For this review, take the finished solid that the model builds, in its own axes (mm). A direction names the side the tool comes from. Coordinates: 2 decimals unless noted, no trailing zeros. Loops run counter-clockwise (first coordinate to the right, second up) from the corner with the lowest first, then second, coordinate; pieces in that order, holes last. Notation, with made-up numbers: (10, 14.25) - (16, 14.25) arc R12 ccw to (16, 23.25) - close; hole circle Ø5 at (-13, -8). An arc over 180 degrees is marked (long way). Answer as a JSON object with one key per item and string values. Group by question number.
Item 1: To check wall thickness, follow line 1 (X direction, y = -18.5, z = 2.5); line 2 (Y direction, x = 21.5, z = -3); line 3 (Y direction, x = 129, z = -10.75). State the ranges of each line that lie inside material, in increasing order.
Item 2: We need section B-B (x = 85.5). Give the boundary of the cut face in (y, z).
Item 3: Clearance check with flat-ended pins moving along their axes: pin 1 (1.5 mm diameter, centred on y = -7, z = -0.5, fed in from +X); pin 2 (6 mm diameter, centred on y = -2, z = 3.5, fed in from -X); pin 3 (5 mm diameter, centred on x = 73.5, y = -7, fed in from -Z); pin 4 (11 mm diameter, centred on x = 49.5, z = 1, fed in from -Y). State where each tip first meets the part, or that it passes through.
Item 4: We need section A-A (y = 0). Give the boundary of the cut face in (x, z).
Item 5: Mouldability with a two-part tool opening along Y and no side actions: class faces 1 (the flat face through (187, 5, 0)), 2 (the cylindrical face through (169.002, -4.507, -0.176)), 3 (the flat face through (193, 4, 0)) as released by +Y, released by -Y, zero draft, split by the parting line, or undercut.
Item 6: We need section C-C (x = 282.5). Give the boundary of the cut face in (y, z), then the cut area to 3 significant figures.
Item 7: Tool access review of faces 4 (the cylindrical face through (370.998, -4.507, 0.176)), 5 (the cylindrical face through (193, 0, -14)), 6 (the cylindrical face through (187, 0, 15)): name each direction out of +Z, -Z, +X, -X, +Y, -Y from which nothing blocks a thin tool from reaching the whole face with its end or side.
from build123d import *

# Parameters (mm, degrees)
EXTRUDE_1_DEPTH          = 380
CUT_EXTRUDE_1_DEPTH      = 0.5
SKETCH_3_W               = 12
SKETCH_3_H               = 8
EXTRUDE_2_DEPTH          = 20
FILLET_1_R               = 6
CUT_EXTRUDE_2_DEPTH      = 382.084308257
CUT_EXTRUDE_2_DEPTH_BACK = 382.084308257
CUT_EXTRUDE_3_DEPTH      = 9
CUT_EXTRUDE_4_DEPTH      = 382.262704706
CUT_EXTRUDE_4_DEPTH_BACK = 382.262704706
SKETCH_6_R               = 2
HOLE_WIZARD_1_64_1_D     = 1.5113
HOLE_WIZARD_1_64_1_DEPTH = 5.69
HOLE_WIZARD_1_64_1_TIP   = 0.454040327


with BuildPart() as part:
    # 草图1 → 凸台-拉伸1 (new body)
    with BuildSketch(Plane(origin=(0, 0, 0), x_dir=(0, 0, -1), z_dir=(1, 0, 0))):
        with BuildLine():
            Line((10, -5), (-10, -5))
            ThreePointArc((-10, -5), (-15, 0), (-10, 5))
            Line((-10, 5), (10, 5))
            ThreePointArc((10, 5), (15, 0), (10, -5))
        make_face()
    extrude(amount=EXTRUDE_1_DEPTH)

    # 草图2 → 切除-拉伸1 (cut)
    with BuildSketch(Plane.XZ.offset(5)):
        with BuildLine():
            Line((73, -5), (43, -5))
            ThreePointArc((43, -5), (38, 0), (43, 5))
            Line((43, 5), (73, 5))
            ThreePointArc((73, 5), (78, 0), (73, -5))
        make_face()
    extrude(amount=-CUT_EXTRUDE_1_DEPTH, mode=Mode.SUBTRACT)

    # 草图3 → 凸台-拉伸2 (add)
    with BuildSketch(Plane.XZ.offset(4.5)):
        with Locations((58, 0)):
            Rectangle(SKETCH_3_W, SKETCH_3_H)
    extrude(amount=EXTRUDE_2_DEPTH)

    # 圆角1
    fillet_1_edges = [part.edges().sort_by_distance(p)[0] for p in [
        (64, -24.5, 0),
        (52, -24.5, 0),
    ]]
    fillet(fillet_1_edges, radius=FILLET_1_R - 0.0001)  # a hair under: the kernel refuses the full size

    # 草图4 → 切除-拉伸2 (cut, two sides: drawn at the far end of the back side and taken through both)
    with BuildSketch(Plane.ZY.offset(-CUT_EXTRUDE_2_DEPTH_BACK)):
        with BuildLine():
            Line((-10, -4), (10, -4))
            ThreePointArc((10, -4), (14, 0), (10, 4))
            Line((10, 4), (-10, 4))
            ThreePointArc((-10, 4), (-14, 0), (-10, -4))
        make_face()
    extrude(amount=CUT_EXTRUDE_2_DEPTH + CUT_EXTRUDE_2_DEPTH_BACK, mode=Mode.SUBTRACT)

    # 草图5 → 切除-拉伸3 (cut)
    with BuildSketch(Plane.XZ.offset(5)):
        with BuildLine():
            Line((363, -8), (177, -8))
            ThreePointArc((177, -8), (169, 0), (177, 8))
            Line((177, 8), (363, 8))
            ThreePointArc((363, 8), (371, 0), (363, -8))
        make_face()
    extrude(amount=-CUT_EXTRUDE_3_DEPTH, mode=Mode.SUBTRACT)

    # 草图6 → 切除-拉伸4 (cut, two sides: drawn at the far end of the back side and taken through both)
    with BuildSketch(Plane.XY.offset(4).offset(-CUT_EXTRUDE_4_DEPTH_BACK)):
        with Locations((58, -18.5)):
            Circle(SKETCH_6_R)
    extrude(amount=CUT_EXTRUDE_4_DEPTH + CUT_EXTRUDE_4_DEPTH_BACK, mode=Mode.SUBTRACT)

    # #1-64 螺纹孔1
    with Locations(Plane(origin=(0, -4.5, 0), x_dir=(-1, 0, 0), z_dir=(0, -1, 0))):
        with Locations((-43, 0), (-73, 0)):
            Hole(HOLE_WIZARD_1_64_1_D / 2, depth=HOLE_WIZARD_1_64_1_DEPTH)
            with Locations((0, 0, -(HOLE_WIZARD_1_64_1_DEPTH + HOLE_WIZARD_1_64_1_TIP / 2))):  # 118° drill point
                Cone(0, HOLE_WIZARD_1_64_1_D / 2, HOLE_WIZARD_1_64_1_TIP, mode=Mode.SUBTRACT)


solid = part.part
Check sheet entries:
{
 "1": {"line 1": "x = 52 to 56, 60 to 64", "line 2": "y = -5 to -4, 4 to 5", "line 3": "y = -4.94 to -3.93, 3.93 to 4.94"},
 "2": {"outline": "(-5, -10) arc R5 ccw to (5, -10) - (5, 10) arc R5 ccw to (-5, 10) - close; hole (-4, -10) arc R4 ccw to (4, -10) - (4, 10) arc R4 ccw to (-4, 10) - close"},
 "3": {"pin 1": "stops at x = 64", "pin 2": "stops at x = 0", "pin 3": "stops at z = -12.18", "pin 4": "stops at y = -23.7"},
 "4": {"outline": "(0, -15) - (380, -15) - (380, -14) - (0, -14) - close; (0, 14) - (380, 14) - (380, 15) - (0, 15) - close"},
 "5": {"face 1": "released by +Y", "face 2": "zero draft", "face 3": "undercut"},
 "6": {"outline": "(-5, -10) arc R5 ccw to (5, -10) - (5, 10) arc R5 ccw to (-5, 10) - (-5, 8) - (-4, 8) - (-4, 10) arc R4 cw to (4, 10) - (4, -10) arc R4 cw to (-4, -10) - (-4, -8) - (-5, -8) - close", "area": "52.3 mm2"},
 "7": {"face 4": "-Y", "face 5": "+X, -X", "face 6": "+Z, +X, -X"}
}
